```python
from build123d import *

# Parameters (mm, degrees)
EXTRUDE_2_DEPTH = 1
SKETCH_4_R      = 11
SKETCH_4_R_2    = 1.5
EXTRUDE_3_DEPTH = 1
EXTRUDE_4_DEPTH = 1
EXTRUDE_5_DEPTH = 1


with BuildPart() as part:
    # 草图3 → 凸台-拉伸2 (new body)
    with BuildSketch(Plane(origin=(0, 0, 0), x_dir=(1, 0, 0), z_dir=(0, 1, 0))):
        Polygon((-25, -20.5), (-20, -25.5), (20, -25.5), (25, -20.5), (25, 25.5), (-25, 25.5), align=None)
        with BuildLine():
            Line((-12.85, 17.5), (-12.85, -12.2))
            ThreePointArc((-12.85, -12.2), (-15, -14.35), (-17.15, -12.2))
            Line((-17.15, -12.2), (-17.15, 17.5))
            ThreePointArc((-17.15, 17.5), (-15, 19.65), (-12.85, 17.5))
        make_face(mode=Mode.SUBTRACT)
        with BuildLine():
            Line((17.15, 17.5), (17.15, -12.2))
            ThreePointArc((17.15, -12.2), (15, -14.35), (12.85, -12.2))
            Line((12.85, -12.2), (12.85, 17.5))
            ThreePointArc((12.85, 17.5), (15, 19.65), (17.15, 17.5))
        make_face(mode=Mode.SUBTRACT)
    extrude(amount=EXTRUDE_2_DEPTH)

    # 草图4 → 凸台-拉伸3 (add)
    with BuildSketch(Plane(origin=(0, 0, -25.5), x_dir=(-1, 0, 0), z_dir=(0, 0, -1))):
        Polygon((-20, 51), (20, 51), (25, 46), (25, 0), (-25, 0), (-25, 46), align=None)
        with Locations((0, 30)):
            Circle(SKETCH_4_R, mode=Mode.SUBTRACT)
        with Locations((-15.5, 45.5)):
            Circle(SKETCH_4_R_2, mode=Mode.SUBTRACT)
        with Locations((15.5, 45.5)):
            Circle(SKETCH_4_R_2, mode=Mode.SUBTRACT)
        with Locations((15.5, 14.5)):
            Circle(SKETCH_4_R_2, mode=Mode.SUBTRACT)
        with Locations((-15.5, 14.5)):
            Circle(SKETCH_4_R_2, mode=Mode.SUBTRACT)
    extrude(amount=-EXTRUDE_3_DEPTH)

    # 草图5 → 凸台-拉伸4 (add)
    with BuildSketch(Plane.ZY.offset(25)):
        Polygon((-25.5, 20), (-25.5, 0), (-5.5, 0), align=None)
    extrude(amount=-EXTRUDE_4_DEPTH)

    # 草图6 → 凸台-拉伸5 (add)
    with BuildSketch(Plane(origin=(25, 0, 0), x_dir=(0, 0, -1), z_dir=(1, 0, 0))):
        Polygon((25.5, 20), (25.5, 0), (5.5, 0), align=None)
    extrude(amount=-EXTRUDE_5_DEPTH)


solid = part.part
```
Can you work these out from the model? Positions are in its coordinate system, mm. A direction names the side the tool comes from. Coordinates: 2 decimals unless noted, no trailing zeros. Write each loop counter-clockwise with the first axis right and the second up, starting at its lowest first coordinate (ties: lowest second). Pieces come first, ordered by that corner, then holes. Notation, with made-up numbers: M 83,47 L 140,47 A24 cw 140,82 Z; hole C 32,22.5 d10. An arc over 180 degrees is marked long. Write item = value, one per line. Start each with the question number.
Q1. If I drill on L1, parallel to Y at x = 0, z = -25.25; L2, parallel to Z at x = -16.5, y = 24; L3, parallel to Y at x = -19, z = 10, over which ranges is the centre line in solid material (lowest first)? Write a range as [from, to].
Q2. If we section it at C-C, the plane z = 6: Write out the boundary of the cut face in (x, y).
Q3. On a 3-axis mill with a long thin cutter (end or side, diameter ignored), from which of +Z, -Z, +X, -X, +Y, -Y can I reach the whole of each face in a straight line? I mean faces 5 (the face through (-22.5, 0.5, 23)), 6 (the face through (15.05, 0.49, 14.35)), 7 (the face through (24, 6, -20)). Say none if no direction works.
Q4. If we section it at D-D, the plane y = 30: Write out the boundary of the cut face in (x, z), then the cut area to 3 significant figures.
Q5. If we section it at B-B, the plane y = 14.5: Write out the boundary of the cut face in (x, z), then the cut area to 3 significant figures.
Q6. If we section it at A-A, the plane x = 0: Write out the boundary of the cut face in (y, z), then the cut area to 3 significant figures.
Q7. Thinking about a two-plate mould opening in Z: for faces 1 (the face through (14.95, 0.49, -19.65)), 2 (the face through (-14.95, 0.49, 14.35)), 3 (the face through (2.38, 19.26, -25.01)), 4 (the face through (0, 15, -24.5)), which applies, released by +Z, released by -Z, zero draft, split by the parting line, or undercut?
Q8. I'm going to push flat-ended pins straight in: pin 1 (1.5 mm diameter, centred on x = 13.5, z = 2, fed in from -Y); pin 2 (3 mm diameter, centred on x = -5.5, z = -19.5, fed in from +Y); pin 3 (25 mm diameter, centred on x = 11, y = 19.5, fed in from +Z). Where does each tip first touch, or does it pass through?
Check sheet entries:
q1.L1 = [0, 19], [41, 51]
q1.L2 = [-25.5, -24.5]
q1.L3 = [0, 1]
q2.outline = M -25,0 L -17.15,0 L -17.15,1 L -25,1 Z; M -12.85,0 L 12.85,0 L 12.85,1 L -12.85,1 Z; M 17.15,0 L 25,0 L 25,1 L 17.15,1 Z
q3.face_5 = +Z, -X, +Y, -Y
q3.face_6 = +Y, -Y
q3.face_7 = +Z, +Y
q4.outline = M -25,-25.5 L -11,-25.5 L -11,-24.5 L -25,-24.5 Z; M 11,-25.5 L 25,-25.5 L 25,-24.5 L 11,-24.5 Z
q4.area = 28.0 mm²
q5.outline = M -25,-25.5 L -17,-25.5 L -17,-24.5 L -24,-24.5 L -24,-20 L -25,-20 Z; M -14,-25.5 L 14,-25.5 L 14,-24.5 L -14,-24.5 Z; M 17,-25.5 L 25,-25.5 L 25,-20 L 24,-20 L 24,-24.5 L 17,-24.5 Z
q5.area = 53.0 mm²
q6.outline = M 0,-25.5 L 19,-25.5 L 19,-24.5 L 1,-24.5 L 1,25.5 L 0,25.5 Z; M 41,-25.5 L 51,-25.5 L 51,-24.5 L 41,-24.5 Z
q6.area = 79.0 mm²
q7.face_1 = undercut
q7.face_2 = undercut
q7.face_3 = zero draft
q7.face_4 = released by +Z
q8.pin_1 = 0
q8.pin_2 = 1
q8.pin_3 = -24.5
